Could you check a few things on this model? Use its own coordinates, in mm. A direction names the side the tool comes from. Coordinates: 2 decimals unless noted, no trailing zeros. Write each loop counter-clockwise with the first axis right and the second up, starting at its lowest first coordinate (ties: lowest second). Pieces come first, ordered by that corner, then holes.
Item 1: I want a section at C-C on x = -46. Please give me the cut outline in (y, z), then the cut area to 3 significant figures.
Item 2: Which directions (+Z, -Z, +X, -X, +Y, -Y) give clear straight access to the entire face, cutting with the end or side of a thin tool? Please do faces 5 (the flat face through (-12.139, -49.083, -115.976)), 6 (the flat face through (-40.906, -49, -96)), 7 (the flat face through (-55, -49, -111.343)).
Item 3: For P1, Ø5, axis at y = -74, z = -130.5, coming from the +X side; P2, Ø5, axis at y = -33.5, z = -103, coming from the +X side; P3, Ø6.5, axis at x = -46, y = -36.5, coming from the -Z side, each with a flat end and sliding along its axis, tell me the tip position at first contact or that it passes through.
Item 4: I want a section at A-A on z = -78. Please give me the cut outline in (x, y), then the cut area to 3 significant figures.
Item 5: If I drill on probe 1 along X at (y, z) = (-39.5, -85); probe 2 along X at (y, z) = (-75, -114.5); probe 3 along Z at (x, y) = (-45, -77.5), over which ranges is the centre line in solid material (lowest first)?
Item 6: I want a section at D-D on z = -112.5. Please give me the cut outline in (x, y), then the cut area to 3 significant figures.
Item 7: Thinking about a two-plate mould opening in X: for faces 1 (the flat face through (-39, -99.56, -103)), 2 (the cylindrical face through (-18.368, -49.083, -141.503)), 3 (the flat face through (-53.476, -49, -89)), 4 (the flat face through (-47, -49, -65.65)), which applies, +X half, -X half, draft (parallel to the pull), parting line (faces both ways), or undercut?
from build123d import *

# Parameters (mm, degrees)
F1_DEPTH = 99.56


# Not quite as in the source:
# - the program builds the solid bodies; features that only make, move or delete a surface that nothing else refers to are left out


with BuildPart() as f1:
    # F0 (on Front) → F1 (new body)
    with BuildSketch(Plane.XZ):
        with BuildLine():
            Line((-53.4761890293, -65.6504866451), (-40.9061890293, -65.6504866451))
            Line((-40.9061890293, -65.6504866451), (-40.9061890293, -127.2904866451))
            ThreePointArc((-40.9061890293, -127.2904866451), (-17.9599684542, -141.3452802415), (-11.0695237566, -115.3339743614))
            Line((-11.0695237566, -115.3339743614), (-13.2391586559, -116.635352248))
            ThreePointArc((-13.2391586559, -116.635352248), (-18.5765544792, -138.8900687432), (-38.3761890293, -127.4124961715))
            Line((-38.3761890293, -127.4124961715), (-38.3761890293, -63.1204866451))
            Line((-38.3761890293, -63.1204866451), (-56.0061890293, -63.1204866451))
            Line((-56.0061890293, -63.1204866451), (-56.0061890293, -111.3434480185))
            Line((-56.0061890293, -111.3434480185), (-53.4761890293, -111.3434480185))
            Line((-53.4761890293, -111.3434480185), (-53.4761890293, -65.6504866451))
        make_face()
    extrude(amount=F1_DEPTH)


solid = f1.part
Response values:
1. outline: (-99.56, -65.65) - (0, -65.65) - (0, -63.12) - (-99.56, -63.12) - close
1. area: 252 mm2
2. face 5: +Z, +Y, -Y
2. face 6: -Z, +Y, -Y
2. face 7: -Z, -X, +Y, -Y
3. P1: stops at x = -7.57
3. P2: stops at x = -38.38
3. P3: stops at z = -65.65
4. outline: (-56.01, -99.56) - (-53.48, -99.56) - (-53.48, 0) - (-56.01, 0) - close; (-40.91, -99.56) - (-38.38, -99.56) - (-38.38, 0) - (-40.91, 0) - close
4. area: 504 mm2
5. probe 1: x = -56.01 to -53.48, -40.91 to -38.38
5. probe 2: x = -40.91 to -38.38
5. probe 3: z = -65.65 to -63.12
6. outline: (-40.91, -99.56) - (-38.38, -99.56) - (-38.38, 0) - (-40.91, 0) - close
6. area: 252 mm2
7. face 1: draft
7. face 2: parting line
7. face 3: undercut
7. face 4: undercut
